Work out the finished part from the listing and answer in its coordinate system (mm). Face numbers are marked on the shaded views. A direction names the side the tool comes from. Coordinates: 2 decimals unless noted, no trailing zeros. Order: outer loops, then holes, each group sorted by start corner. A loop starts at its lowest first (then second) coordinate and runs counter-clockwise, first axis right, second up. Notation, with made-up numbers: (6, 71) -> (51, 71) arc R36 ccw to (51, 108) -> close; hole circle Ø4 at (11, 76). An arc over 180 degrees is marked (long way). Use one line per item in the form item = value.
from build123d import *

# Parameters (mm, degrees)
F0_R     = 19
F1_DEPTH = 4
F2_W     = 3
F2_H     = 15
F3_DEPTH = 13
F2_W_2   = 4
F4_DEPTH = 13
F5_R     = 5
F6_DEPTH = 10


with BuildPart() as f1:
    # F0 (on Top) → F1 (new body)
    with BuildSketch(Plane.XY):
        with BuildLine():
            Line((-41.5, -7.5), (-21.2132034356, -7.5))
            ThreePointArc((-21.2132034356, -7.5), (0, -22.5), (21.2132034356, -7.5))
            Line((21.2132034356, -7.5), (41.5, -7.5))
            Line((41.5, -7.5), (41.5, 7.5))
            Line((41.5, 7.5), (21.2132034356, 7.5))
            ThreePointArc((21.2132034356, 7.5), (15.9099025767, 15.9099025767), (7.5, 21.2132034356))
            Line((7.5, 21.2132034356), (7.238372093, 41.5))
            Line((7.238372093, 41.5), (-7.5, 41.5))
            Line((-7.5, 41.5), (-7.5, 21.2132034356))
            ThreePointArc((-7.5, 21.2132034356), (-15.9099025767, 15.9099025767), (-21.2132034356, 7.5))
            Line((-21.2132034356, 7.5), (-41.5, 7.5))
            Line((-41.5, 7.5), (-41.5, -7.5))
        make_face()
        Circle(F0_R, mode=Mode.SUBTRACT)
    extrude(amount=F1_DEPTH)

    # F2 (on face) → F3 (join)
    with BuildSketch(Plane.XY.offset(4)):
        Polygon((7.238372093, 41.5), (7.2770614799, 38.5), (7.2770614799, 41.5), align=None)
        with Locations((-40, 0)):
            Rectangle(F2_W, F2_H)
        with Locations((40, 0)):
            Rectangle(F2_W, F2_H)
        Polygon((-7.5, 41.5), (-7.5, 38.5), (7.2770614799, 38.5), (7.238372093, 41.5), align=None)
    extrude(amount=F3_DEPTH)

    # F2 (on face) → F4 (join)
    with BuildSketch(Plane.XY.offset(4)):
        with Locations((-36.5, 0)):
            Rectangle(F2_W_2, F2_H)
        with Locations((36.5, 0)):
            Rectangle(F2_W_2, F2_H)
        Polygon((-7.5, 38.5), (-7.5, 34.5), (7.3286473291, 34.5), (7.2770614799, 38.5), align=None)
    extrude(amount=F4_DEPTH)

    # F5
    f5_edges = [f1.edges().sort_by_distance(p)[0] for p in [
        (-21.213203, -7.5, 2),
        (21.213203, -7.5, 2),
        (21.213203, 7.5, 2),
        (7.5, 21.213203, 2),
        (-21.213203, 7.5, 2),
        (-7.5, 21.213203, 2),
    ]]
    fillet(f5_edges, radius=F5_R)

    # F2 (on face) → F6 (cut)
    with BuildSketch(Plane.XY.offset(4)):
        Polygon((-7.5, 38.5), (-7.5, 34.5), (7.3286473291, 34.5), (7.2770614799, 38.5), align=None)
        with Locations((-36.5, 0)):
            Rectangle(F2_W_2, F2_H)
        with Locations((36.5, 0)):
            Rectangle(F2_W_2, F2_H)
    extrude(amount=F6_DEPTH, mode=Mode.SUBTRACT)


solid = f1.part
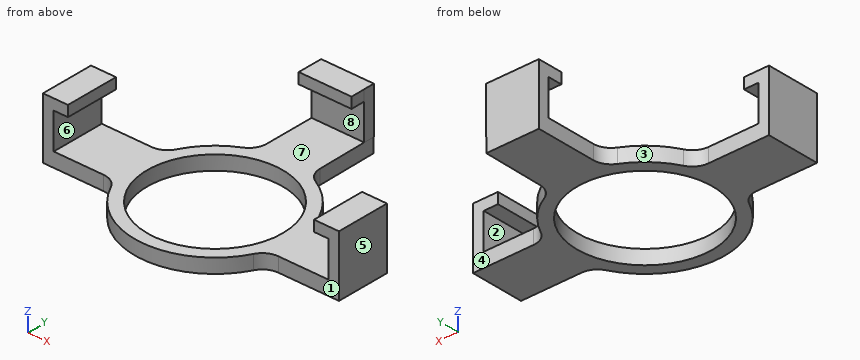
(1) The mould has two halves that part along X. Classify the marked faces 1, 2 and 3: released by +X, released by -X, zero draft, split by the parting line, or undercut.
Data:
face_1 = zero draft
face_2 = undercut
face_3 = released by -X
(2) Section D-D on z = 3 is taken. Write down the section's boundary in (x, y), plus the area to 3 significant figures.
Data:
outline = (-41.5, -7.5) -> (-24.49, -7.5) arc R5 cw to (-20.04, -10.23) arc R22.5 ccw to (20.04, -10.23) arc R5 cw to (24.49, -7.5) -> (41.5, -7.5) -> (41.5, 7.5) -> (24.49, 7.5) arc R5 cw to (20.04, 10.23) arc R22.5 ccw to (10.19, 20.06) arc R5 cw to (7.46, 24.45) -> (7.24, 41.5) -> (-7.5, 41.5) -> (-7.5, 24.49) arc R5 cw to (-10.23, 20.04) arc R22.5 ccw to (-20.04, 10.23) arc R5 cw to (-24.49, 7.5) -> (-41.5, 7.5) -> close; hole circle Ø38 at (0, 0)
area = 1,340 mm²
(3) Section C-C on x = 0 is taken. Write down the section's boundary in (y, z), plus the area to 3 significant figures.
Data:
outline = (-22.5, 0) -> (-19, 0) -> (-19, 4) -> (-22.5, 4) -> close; (19, 0) -> (41.5, 0) -> (41.5, 17) -> (34.5, 17) -> (34.5, 14) -> (38.5, 14) -> (38.5, 4) -> (19, 4) -> close
area = 155 mm²
(4) Each of these flat-tipped pins is pushed along its axis until it touches: P1, Ø2, axis at x = -16, z = 3.5, coming from the -Y side; P2, Ø2.5, axis at x = -1, z = 16, coming from the -Y side; P3, Ø2, axis at x = -36.5, y = 2, coming from the -Z side; P4, Ø3.5, axis at y = 39.5, z = 12.5, coming from the +X side. Where does it stop, or does it pass through?
Data:
P1 = -16.77
P2 = 34.5
P3 = 0
P4 = 7.28
(5) Straight lines are drawn through the part: line 1 along X through (y, z) = (1, 16.5); line 2 along Z through (x, y) = (6.5, 21); line 3 along Y through (x, z) = (29.5, 1.25). For each, find the intervals that lie inside material, in ascending order.
Data:
line_1 = -41.5 to -34.5, 34.5 to 41.5
line_2 = 0 to 4
line_3 = -7.5 to 7.5
(6) Section B-B on z = 10 is taken. Write down the section's boundary in (x, y), plus the area to 3 significant figures.
Data:
outline = (-41.5, -7.5) -> (-38.5, -7.5) -> (-38.5, 7.5) -> (-41.5, 7.5) -> close; (-7.5, 38.5) -> (7.28, 38.5) -> (7.28, 41.5) -> (-7.5, 41.5) -> close; (38.5, -7.5) -> (41.5, -7.5) -> (41.5, 7.5) -> (38.5, 7.5) -> close
area = 134 mm²
(7) Which of the six approach directions +Z, -Z, +X, -X, +Y, -Y give full straight-line access (tool end or side, diameter ignored) to the marked faces 4, 5, 6, 7 and 8?
Data:
face_4 = +Z, -Z, +X, +Y
face_5 = +Z, -Z, +X, +Y, -Y
face_6 = +Y, -Y
face_7 = -Y
face_8 = +X, -X, -Y
(8) Section A-A on y = 0 is taken. Write down the section's boundary in (x, z), plus the area to 3 significant figures.
Data:
outline = (-41.5, 0) -> (-19, 0) -> (-19, 4) -> (-38.5, 4) -> (-38.5, 14) -> (-34.5, 14) -> (-34.5, 17) -> (-41.5, 17) -> close; (19, 0) -> (41.5, 0) -> (41.5, 17) -> (34.5, 17) -> (34.5, 14) -> (38.5, 14) -> (38.5, 4) -> (19, 4) -> close
area = 282 mm²
